```python
from build123d import *

# Parameters (mm, degrees)
BOSS_EXTRUDE1_DEPTH = 12.7
SKETCH2_R           = 3.175
CUT_EXTRUDE1_DEPTH  = 12.7


with BuildPart() as part:
    # Sketch1 → Boss-Extrude1 (new body)
    with BuildSketch(Plane.YZ):
        with BuildLine():
            Line((-12.7, 0), (-12.7, 152.4))
            ThreePointArc((-12.7, 152.4), (0, 165.1), (12.7, 152.4))
            Line((12.7, 152.4), (12.7, 0))
            ThreePointArc((12.7, 0), (0, -12.7), (-12.7, 0))
        make_face()
    extrude(amount=BOSS_EXTRUDE1_DEPTH)

    # Sketch2 → Cut-Extrude1 (cut)
    with BuildSketch(Plane.YZ.offset(12.7)):
        with Locations(Location((0, 0, 0), (0, 0, 270))):
            Circle(SKETCH2_R)
        with Locations(Location((0, 152.4, 0), (0, 0, 270))):
            Circle(SKETCH2_R)
    extrude(amount=-CUT_EXTRUDE1_DEPTH, mode=Mode.SUBTRACT)


solid = part.part
```
CAD build for the part. Positions are in the model's coordinates, mm. Coordinates: 2 decimals unless noted, no trailing zeros. Write each loop counter-clockwise with the first axis right and the second up, starting at its lowest first coordinate (ties: lowest second). Pieces come first, ordered by that corner, then holes. Notation, with made-up numbers: (85, 56.25) -> (126, 56.25) arc R25 ccw to (126, 94.25) -> close; hole circle Ø5 at (54.5, -8). An arc over 180 degrees is marked (long way). Return JSON: item names as keys, results as strings. Group by question number.
Q1. Cut at D-D, the plane y = 8.75. Give the cut face in (x, z), then the cut area to 3 significant figures.
Q2. Flat gauge pins, fed straight in: pin 1 (6 mm diameter, centred on x = 1.5, y = 6.5, fed in from -Z); pin 2 (4 mm diameter, centred on x = 6.5, y = -2.5, fed in from +Z); pin 3 (2 mm diameter, centred on x = 6, y = -10, fed in from +Z); pin 4 (4 mm diameter, centred on y = 0, z = 0, fed in from +X). Where does each tip first touch, or does it go through?
Q3. Cut at C-C, the plane z = 154. Give the cut face in (x, y).
Q4. Drill centre lines: line 1 (Y direction, x = 3.25, z = 0) (3 decimals); line 2 (Z direction, x = 11.75, y = 1.25); line 3 (Y direction, x = 4.25, z = 151). Where is each one in solid material? Low to high.
Q5. Cut at A-A, the plane y = 0. Give the cut face in (x, z) (3 decimals), then the cut area to 3 significant figures.
Q6. Cut at B-B, the plane x = 9.5. Give the cut face in (y, z) (3 decimals).
Q7. Pull direction Y, two halves, no side cores. Call faces 1 (the face through (12.7, 0, 77)), 2 (the face through (6.261, 0.279, -12.697)), 3 (the face through (6.44, -1.93, 2.52)): released by +Y, released by -Y, zero draft, split by the parting line, or undercut.
Returned:
{
 "1": {"outline": "(0, -9.2) -> (12.7, -9.2) -> (12.7, 161.6) -> (0, 161.6) -> close", "area": "2,170 mm2"},
 "2": {"pin 1": "stops at z = -12.21", "pin 2": "stops at z = 165.09", "pin 3": "stops at z = 161.36", "pin 4": "passes through"},
 "3": {"outline": "(0, -12.6) -> (12.7, -12.6) -> (12.7, -2.74) -> (0, -2.74) -> close; (0, 2.74) -> (12.7, 2.74) -> (12.7, 12.6) -> (0, 12.6) -> close"},
 "4": {"line 1": "y = -12.7 to -3.175, 3.175 to 12.7", "line 2": "z = -12.64 to -2.92, 2.92 to 149.48, 155.32 to 165.04", "line 3": "y = -12.7 to -2.85, 2.85 to 12.7"},
 "5": {"outline": "(0, -12.7) -> (12.7, -12.7) -> (12.7, -3.175) -> (0, -3.175) -> close; (0, 3.175) -> (12.7, 3.175) -> (12.7, 149.225) -> (0, 149.225) -> close; (0, 155.575) -> (12.7, 155.575) -> (12.7, 165.1) -> (0, 165.1) -> close", "area": "2,100 mm2"},
 "6": {"outline": "(-12.7, 0) arc R12.7 ccw to (12.7, 0) -> (12.7, 152.4) arc R12.7 ccw to (-12.7, 152.4) -> close; hole circle Ø6.35 at (0, 0); hole circle Ø6.35 at (0, 152.4)"},
 "7": {"face 1": "zero draft", "face 2": "split by the parting line", "face 3": "undercut"}
}
